Answer from the drawing. Dimensions are ordinates in mm from the lowest x, y and z of the part. Coordinates: 2 decimals unless noted, no trailing zeros. Write each loop counter-clockwise with the first axis right and the second up, starting at its lowest first coordinate (ties: lowest second). Pieces come first, ordered by that corner, then holes.
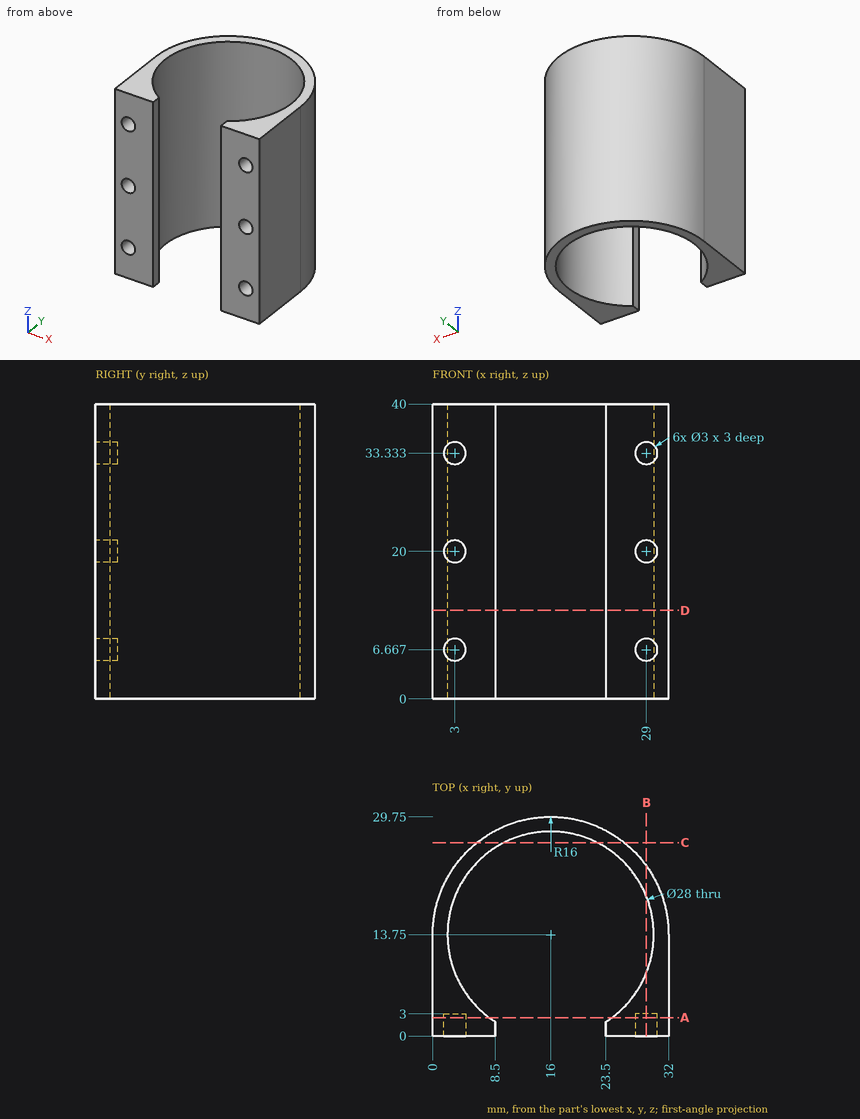
(1) Section D-D, the plane z = 12 is taken. Write down the section's boundary in (x, y).
(2) Each of these flat-tipped pins is pushed along its axis until it touches: pin 1 (2 mm diameter, centred on y = 19.5, z = 18.5, fed in from -X); pin 2 (4 mm diameter, centred on x = 5.5, z = 29, fed in from +Y) (1 decimal); pin 3 (5 mm diameter, centred on x = 29, z = 33.33, fed in from +Y); pin 4 (1.5 mm diameter, centred on x = 23, y = 4.5, fed in from +Z). Where does it stop, or does it pass through?
(3) Find the intervals of material crossed by probe 1 along Z at (x, y) = (29, 2.2); probe 2 along X at (y, z) = (16.25, 35) (1 decimal); probe 3 along X at (y, z) = (3, 27), in increasing order.
(4) Section C-C, the plane y = 26.25 is taken. Write down the section's boundary in (x, z) (1 decimal).
(5) Section A-A, the plane y = 2.5 is taken. Write down the section's boundary in (x, z), plus the area to 3 significant figures.
(6) Section B-B, the plane x = 29 is taken. Write down the section's boundary in (y, z).
Solution:
1. outline: (0, 0) - (8.5, 0) - (8.5, 1.93) arc R14 cw (long way) to (23.5, 1.93) - (23.5, 0) - (32, 0) - (32, 13.75) arc R16 ccw to (0, 13.75) - close
2. pin 1: stops at x = 0.72
2. pin 2: stops at y = 27.3
2. pin 3: stops at y = 25.82
2. pin 4: passes through
3. probe 1: z = 0 to 5.17, 8.17 to 18.5, 21.5 to 31.83, 34.83 to 40
3. probe 2: x = 0.2 to 2.2, 29.8 to 31.8
3. probe 3: x = 0 to 7.03, 24.97 to 32
4. outline: (6, 0) - (9.7, 0) - (9.7, 40) - (6, 40) - close; (22.3, 0) - (26, 0) - (26, 40) - (22.3, 40) - close
5. outline: (0, 0) - (7.67, 0) - (7.67, 40) - (0, 40) - close; (24.33, 0) - (32, 0) - (32, 40) - (24.33, 40) - close; hole circle Ø3 at (3, 6.67); hole circle Ø3 at (3, 20); hole circle Ø3 at (3, 33.33); hole circle Ø3 at (29, 6.67); hole circle Ø3 at (29, 20); hole circle Ø3 at (29, 33.33)
5. area: 571 mm2
6. outline: (0, 0) - (8.55, 0) - (8.55, 40) - (0, 40) - (0, 34.83) - (3, 34.83) - (3, 31.83) - (0, 31.83) - (0, 21.5) - (3, 21.5) - (3, 18.5) - (0, 18.5) - (0, 8.17) - (3, 8.17) - (3, 5.17) - (0, 5.17) - close; (18.95, 0) - (23.08, 0) - (23.08, 40) - (18.95, 40) - close
